CAD build for the part. Positions are in the model's coordinates, mm. A direction names the side the tool comes from. Round coordinates to 2 decimals unless told otherwise and drop trailing zeros. Order: outer loops, then holes, each group sorted by start corner. A loop starts at its lowest first (then second) coordinate and runs counter-clockwise, first axis right, second up. Notation, with made-up numbers: (-23.75, 80) -> (-15.75, 80) arc R21 ccw to (-15.75, 104) -> close; hole circle Ø3 at (-20, 11). An arc over 180 degrees is marked (long way). Answer as CSV lines item,"result". Start each with the question number.
from build123d import *

# Parameters (mm, degrees)
F_3_4_16_TAPPED_HOLE1_REACH  = 167.74
F_3_4_16_TAPPED_HOLE1_BORE_R = 8.73125


with BuildPart() as part:
    # Sketch1 → Revolve1 (revolve)
    with BuildSketch(Plane.XY, mode=Mode.PRIVATE) as revolve1_sk:
        Polygon((-127, 0), (-127, 47.625), (127, 47.625), (127, 38.1), (-120.65, 38.1), (-120.65, 0), align=None)
    revolve(revolve1_sk.sketch.rotate(Axis((-127, 0, 0), (1, 0, 0)), 90), axis=Axis((-127, 0, 0), (1, 0, 0)))

    # 3/4-16 Tapped Hole1 bore → 3/4-16 Tapped Hole1 (cut, up to next)
    with BuildSketch(Plane(origin=(0, 47.625, 0), x_dir=(1, 0, 0), z_dir=(0, 1, 0)), mode=Mode.PRIVATE) as f_3_4_16_tapped_hole1_sk1:
        with Locations((-88.9, 0)):
            Circle(F_3_4_16_TAPPED_HOLE1_BORE_R)
    f_3_4_16_tapped_hole1_tool1 = extrude(f_3_4_16_tapped_hole1_sk1.sketch, amount=-F_3_4_16_TAPPED_HOLE1_REACH, mode=Mode.PRIVATE) & part.part
    # 3/4-16 Tapped Hole1 bore → 3/4-16 Tapped Hole1 (cut, up to next)
    with BuildSketch(Plane(origin=(0, 47.625, 0), x_dir=(1, 0, 0), z_dir=(0, 1, 0)), mode=Mode.PRIVATE) as f_3_4_16_tapped_hole1_sk2:
        with Locations((88.9, 0)):
            Circle(F_3_4_16_TAPPED_HOLE1_BORE_R)
    f_3_4_16_tapped_hole1_tool2 = extrude(f_3_4_16_tapped_hole1_sk2.sketch, amount=-F_3_4_16_TAPPED_HOLE1_REACH, mode=Mode.PRIVATE) & part.part
    add(f_3_4_16_tapped_hole1_tool1.solids().sort_by_distance((-88.9, 47.625, 0))[0], mode=Mode.SUBTRACT)
    add(f_3_4_16_tapped_hole1_tool2.solids().sort_by_distance((88.9, 47.625, 0))[0], mode=Mode.SUBTRACT)


solid = part.part
Item 1: Band-saw the part on D-D, the plane y = -30.5. Give the cut face in (x, z), and give its area (3 significant figures).
Item 2: Pin check, flat tips, straight feed: pin 1 (4 mm diameter, centred on x = -99, y = 24, fed in from -Z); pin 2 (2 mm diameter, centred on x = 42, y = 31.5, fed in from +Z); pin 3 (12 mm diameter, centred on x = 72.5, z = 10.5, fed in from +Y). Stop position of each tip, or through.
Item 3: Band-saw the part on A-A, the plane z = 0. Give the cut face in (x, y) (3 decimals), and give its area (3 significant figures).
Item 4: Probe line 1 (X direction, y = 40, z = 0); line 2 (X direction, y = 41, z = -5.5); line 3 (Z direction, x = -2, y = 2). List the from-to ranges inside material, lowest first.
Item 5: Band-saw the part on B-B, the plane y = 41. Give the cut face in (x, z).
Item 6: Mould opens along Y. For faces 3 (the cylindrical face through (1.778, 46.492, -10.324)), 4 (the cylindrical face through (80.177, 42.429, -0.384)), 5 (the flat face through (-120.65, -1, -1)), 6 (the cylindrical face through (1.441, 37.194, -8.259)) say: released by +Y, released by -Y, zero draft, split by the parting line, or undercut.
Item 7: Band-saw the part on C-C, the plane x = -8. Give the cut face in (y, z) (3 decimals), and give its area (3 significant figures).
Item 8: Tool access for faces 1 (the flat face through (-127, -1, 1)), 2 (the cylindrical face through (-97.623, 42.429, -0.384)): list every direction of +Z, -Z, +X, -X, +Y, -Y with a clear straight run to the whole face (end or side of a thin tool).
Values:
1,outline,"(-127, -36.58) -> (127, -36.58) -> (127, -22.83) -> (-120.65, -22.83) -> (-120.65, 22.83) -> (127, 22.83) -> (127, 36.58) -> (-127, 36.58) -> close"
1,area,"7,270 mm²"
2,pin 1,"z = -42.24"
2,pin 2,"z = 36.58"
2,pin 3,"y = 47.41"
3,outline,"(-127, -47.625) -> (127, -47.625) -> (127, -38.1) -> (-120.65, -38.1) -> (-120.65, 38.1) -> (-97.631, 38.1) -> (-97.631, 47.625) -> (-127, 47.625) -> close; (-80.169, 38.1) -> (80.169, 38.1) -> (80.169, 47.625) -> (-80.169, 47.625) -> close; (97.631, 38.1) -> (127, 38.1) -> (127, 47.625) -> (97.631, 47.625) -> close"
3,area,"4,990 mm²"
4,line 1,"-127 to -97.63, -80.17 to 80.17, 97.63 to 127"
4,line 2,"-127 to -95.68, -82.12 to 82.12, 95.68 to 127"
4,line 3,"-47.58 to -38.05, 38.05 to 47.58"
5,outline,"(-127, -24.23) -> (127, -24.23) -> (127, 24.23) -> (-127, 24.23) -> close; hole circle Ø17.46 at (-88.9, 0); hole circle Ø17.46 at (88.9, 0)"
6,face 3,"split by the parting line"
6,face 4,"zero draft"
6,face 5,"undercut"
6,face 6,"undercut"
7,outline,"circle Ø95.25 at (0, 0); hole circle Ø76.2 at (0, 0)"
7,area,"2,570 mm²"
8,face 1,"+Z, -Z, -X, +Y, -Y"
8,face 2,"+Y"
